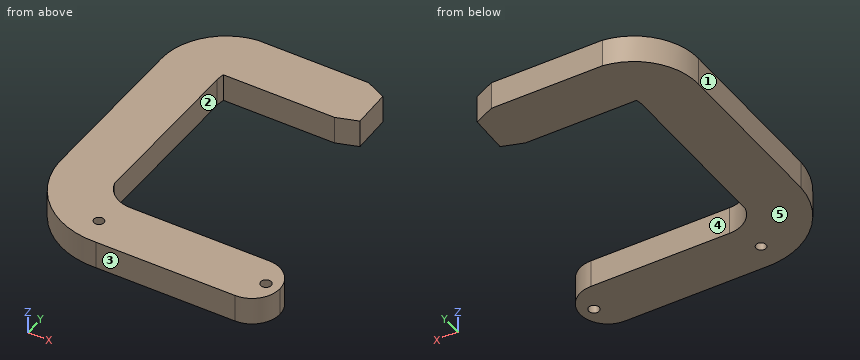
from build123d import *

# Parameters (mm, degrees)
F0_W     = 20
F0_H     = 60
F0_W_2   = 40
F0_H_2   = 20
F1_DEPTH = 5
F2_R     = 1.9
F3_DEPTH = 26
F4_R     = 1.8
F5_DEPTH = 25


with BuildPart() as f1:
    # F0 (on Top) → F1 (new body, symmetric)
    with BuildSketch(Plane.XY):
        with BuildLine():
            ThreePointArc((30, 0), (27.071068, 7.071068), (20, 10))
            Line((20, 10), (-30, 10))
            Line((-30, 10), (-30, -10))
            Line((-30, -10), (20, -10))
            ThreePointArc((20, -10), (27.071068, -7.071068), (30, 0))
        make_face()
        with BuildLine():
            Line((-30, -10), (-30, 10))
            ThreePointArc((-30, 10), (-36.446695, 12.117762), (-40.381671, 17.645941))
            Line((-40.381671, 17.645941), (-60.381671, 17.645941))
            ThreePointArc((-60.381671, 17.645941), (-50.903472, -2.454966), (-30, -10))
        make_face()
        with Locations((-50.381671, 47.645941)):
            Rectangle(F0_W, F0_H)
        with BuildLine():
            Line((-60.381671, 77.645941), (-40.381671, 77.645941))
            ThreePointArc((-40.381671, 77.645941), (-40.285886, 79.190626), (-40, 80.711644))
            Line((-40, 80.711644), (-40, 100.711644))
            ThreePointArc((-40, 100.711644), (-54.556209, 93.036191), (-60.381671, 77.645941))
        make_face()
        with Locations((-20, 90.711644)):
            Rectangle(F0_W_2, F0_H_2)
        Polygon((0, 100.711644), (0, 80.711644), (7.590995, 83.236875), (7.203378, 97.231508), align=None)
    extrude(amount=F1_DEPTH, both=True)

    # F2 (on face) → F3 (cut)
    with BuildSketch(Plane.XY.offset(5)):
        with Locations((25.055628, -0.060417)):
            Circle(F2_R)
    extrude(amount=-F3_DEPTH, mode=Mode.SUBTRACT)

    # F4 (on face) → F5 (cut)
    with BuildSketch(Plane.XY.offset(5)):
        with Locations((-34.756718, -0.582021)):
            Circle(F4_R)
    extrude(amount=-F5_DEPTH, mode=Mode.SUBTRACT)


solid = f1.part
Verification items for the finished model (mm, model axes). Face numbers are marked on the shaded views. A direction names the side the tool comes from. Coordinates: 2 decimals unless noted, no trailing zeros. Loops run counter-clockwise (first coordinate to the right, second up) from the corner with the lowest first, then second, coordinate; pieces in that order, holes last. Notation, with made-up numbers: (-18.5, 88) -> (5.5, 88) arc R23 ccw to (5.5, 102) -> close; hole circle Ø5 at (-37, 38.25). An arc over 180 degrees is marked (long way). Answer as CSV lines item,"result".
1) Release check for a two-part mould opening along Y. For the marked faces 1, 2 and 3 record: +Y half, -Y half, draft (parallel to the pull), parting line (faces both ways), or undercut.
Found:
face 1,"draft"
face 2,"undercut"
face 3,"-Y half"
2) Tool access check on the marked faces 4 and 5. Record the directions out of +Z, -Z, +X, -X, +Y, -Y that give a thin tool (end or side, any length) a straight path to the whole face; none if there is none.
Found:
face 4,"+Z, -Z, +X"
face 5,"-Z, +X, -X, +Y, -Y"
3) Cross-section at B-B, the plane z = -3.75. Record the cut outline in (x, y), then the cut area to 3 significant figures.
Found:
outline,"(-60.38, 17.65) arc R29.09 ccw to (-30, -10) -> (20, -10) arc R10 ccw to (30, 0) arc R10 ccw to (20, 10) -> (-30, 10) arc R10.87 cw to (-40.38, 17.65) -> (-40.38, 77.65) arc R12.5 cw to (-40, 80.71) -> (0, 80.71) -> (7.59, 83.24) -> (7.2, 97.23) -> (0, 100.71) -> (-40, 100.71) arc R23.24 ccw to (-60.38, 77.65) -> close; hole circle Ø3.6 at (-34.76, -0.58); hole circle Ø3.8 at (25.06, -0.06)"
area,"4,220 mm2"
4) Depth check by flat-ended pin: pin 1 (3 mm diameter, centred on y = 62, z = 0.5, fed in from +X); pin 2 (5 mm diameter, centred on x = 7.5, z = 1.5, fed in from -Y); pin 3 (1.5 mm diameter, centred on y = 85.5, z = -3, fed in from -X). Enter the tip coordinate at first touch or a pass-through.
Found:
pin 1,"stops at x = -40.38"
pin 2,"stops at y = -10"
pin 3,"stops at x = -59.27"
5) Thickness scan on L1, parallel to Y at x = -25, z = 0.5; L2, parallel to X at y = 76.5, z = 4; L3, parallel to Y at x = 9.5, z = 2.75. Record the ranges inside material, lowest first. Write a range as from..to.
Found:
L1,"y = -10..10, 80.71..100.71"
L2,"x = -60.38..-40.38"
L3,"y = -10..10"
6) Cross-section at D-D, the plane x = 17. Record the cut outline in (y, z), then the cut area to 3 significant figures.
Found:
outline,"(-10, -5) -> (10, -5) -> (10, 5) -> (-10, 5) -> close"
area,"200 mm2"
7) Cross-section at C-C, the plane y = 57. Record the cut outline in (x, z).
Found:
outline,"(-60.38, -5) -> (-40.38, -5) -> (-40.38, 5) -> (-60.38, 5) -> close"
8) Cross-section at A-A, the plane x = -9.5. Record the cut outline in (y, z), then the cut area to 3 significant figures.
Found:
outline,"(-10, -5) -> (10, -5) -> (10, 5) -> (-10, 5) -> close; (80.71, -5) -> (100.71, -5) -> (100.71, 5) -> (80.71, 5) -> close"
area,"400 mm2"
